The model under review builds one solid part; all positions refer to its coordinate system, in mm. A direction names the side the tool comes from. Coordinates: 2 decimals unless noted, no trailing zeros. Order: outer loops, then holes, each group sorted by start corner. A loop starts at its lowest first (then second) coordinate and runs counter-clockwise, first axis right, second up. Notation, with made-up numbers: M -30,70 L 18,70 A10 cw 18,75 Z; hole C 65,-30.5 d10. An arc over 180 degrees is marked long. Answer as CSV lines item,"result". Start each with the question number.
Q1. Consider section A-A on x = 18. Write out the cut boundary in (y, z), and give its area (3 significant figures).
Q2. Consider section D-D on y = -18. Write out the cut boundary in (x, z), and give its area (3 significant figures).
Q3. Consider section C-C on z = 13.5. Write out the cut boundary in (x, y).
Q4. The part is to be moulded in two halves that separate along Z. For faces 3 (the face through (0, 4, 29.651)), 4 (the face through (0.444, 5.546, 32.027)), 5 (the face through (0, -5.514, -16)), 6 (the face through (0.444, -12.716, 49.619)), say which applies: +Z half, -Z half, draft (parallel to the pull), parting line (faces both ways), or undercut.
Q5. Consider section B-B on y = -1. Write out the cut boundary in (x, z).
Q6. Wall thickness on L1, parallel to Y at x = -21, z = -14.5; L2, parallel to Y at x = 3, z = 31.5; L3, parallel to Z at x = 14, y = -0.5: over which ranges is each line inside the solid? List them lowest first. Write a range as [from, to].
Q7. Machinability: for faces 1 (the face through (0, -2.573, 13)), 2 (the face through (0, 0, -29.651)), which of the approach directions +Z, -Z, +X, -X, +Y, -Y give a long, thin tool a straight path to every point of the face, cutting with its end or side? Answer none if there is none.
Q8. For P1, Ø1.5, axis at x = -9.5, z = 22.5, coming from the -Y side; P2, Ø1.5, axis at x = -19, y = -24, coming from the -Z side; P3, Ø4, axis at x = -18.5, z = -15, coming from the -Y side, all flat-tipped, find the tip position at first contact; note any pin that passes through.
from build123d import *

# Parameters (mm, degrees)
F1_DEPTH    = 31.75
F2_T1_DEPTH = 89.6282991577
F2_T6_DEPTH = 89.6282991577
F4_DEPTH    = 31.75


# Not quite as in the source:
# - a fillet or chamfer that OpenCascade refuses, or shapes differently, is made with other operations: its cross-section is extruded or revolved along the edge and cut away or added


with BuildPart() as f1:
    # F0 (on Right) → F1 (new body, symmetric)
    with BuildSketch(Plane.YZ):
        Polygon((5.5137062445, 29.6514853835), (-2.5730628986, 29.6514853835), (-2.5730628986, 2.6955895592), (-5.5137062445, 2.6955895592), (-5.5137062445, -29.6514853835), (5.5137062445, -29.6514853835), align=None)
    extrude(amount=F1_DEPTH, both=True)

    # F2: chamfer of 5.08 on 2 edges, made by hand

    # F2_s2 → F2_t1 (cut)
    with BuildSketch(Plane.YZ.offset(-44.8141495789)):
        Polygon((2.5069371014, 29.6514853835), (-2.5730628986, 24.5714853835), (-2.5730628986, 29.6514853835), align=None)
    extrude(amount=F2_T1_DEPTH, mode=Mode.SUBTRACT)


with BuildPart() as f2_tool4:
    # F2_s5 → F2_t6 (new body)
    with BuildSketch(Plane.YZ.offset(-44.8141495789)):
        Polygon((-5.5137062445, -2.3844104408), (-0.4337062445, 2.6955895592), (-5.5137062445, 2.6955895592), align=None)
    extrude(amount=F2_T6_DEPTH)

    split(bisect_by=Plane.XZ.offset(2.5730628986), keep=Keep.TOP)


with BuildPart() as f1_1:
    add(f1.part)

    # F2_t3: cut F2_tool4
    add(f2_tool4.part, mode=Mode.SUBTRACT)

    # F3 (on Right) → F4 (join, symmetric)
    with BuildSketch(Plane.YZ):
        Polygon((5.3522153758, 29.5617226511), (5.411314778, -29.3982010335), (6.4068306237, -29.3982010335), (6.4068306237, 34.8174758255), (6.0373530723, 35.9628349543), (5.3522153758, 36.7688797414), (4.586473573, 37.2525081038), (-30.5093135685, 62.3375996947), (-30.9179358327, 61.7659087381), (4.054645617, 36.7688797414), (4.8554181121, 36.1976027489), (5.3522153758, 35.3252030909), (5.7278168388, 34.3364849687), align=None)
    extrude(amount=F4_DEPTH, both=True)


solid = f1_1.part
Evaluation:
1,outline,"M -30.92,61.77 L 4.05,36.77 L 4.86,36.2 L 5.35,35.33 L 5.73,34.34 L 5.36,29.65 L 2.51,29.65 L -2.57,24.57 L -2.57,0.56 L -5.51,-2.38 L -5.51,-29.65 L 5.51,-29.65 L 5.51,-29.4 L 6.41,-29.4 L 6.41,34.82 L 6.04,35.96 L 5.35,36.77 L 4.59,37.25 L -30.51,62.34 Z"
1,area,"641 mm²"
2,outline,"M -31.75,52.53 L 31.75,52.53 L 31.75,53.4 L -31.75,53.4 Z"
2,area,"54.8 mm²"
3,outline,"M -31.75,-2.57 L 31.75,-2.57 L 31.75,6.41 L -31.75,6.41 Z"
4,face 3,"undercut"
4,face 4,"undercut"
4,face 5,"draft"
4,face 6,"+Z half"
5,outline,"M -31.75,-29.65 L 31.75,-29.65 L 31.75,26.14 L -31.75,26.14 Z; M -31.75,40.38 L 31.75,40.38 L 31.75,41.25 L -31.75,41.25 Z"
6,L1,"y = [-5.51, 6.41]"
6,L2,"y = [5.5, 6.41]"
6,L3,"z = [-29.65, 26.64], [40.02, 40.89]"
7,face 1,"+X, -X, -Y"
7,face 2,"-Z, +X, -X, +Y, -Y"
8,P1,"stops at y = -2.57"
8,P2,"stops at z = 56.29"
8,P3,"stops at y = -5.51"
